The listing builds one solid part. Answer for the finished solid, in the listing's coordinates (mm). A direction names the side the tool comes from. Give positions to 0.01 mm unless a question says otherwise; leave off trailing zeros. Write each loop counter-clockwise with the first axis right and the second up, starting at its lowest first coordinate (ties: lowest second). Pieces come first, ordered by that corner, then holes.
```python
from build123d import *

# Parameters (mm, degrees)
BASPROSKE_W         = 3.175
BASPROSKE_H         = 5.291666667
TOOTHCUT_DEPTH      = 9.129212583
TEETHCUTS_COUNT     = 18
TEETHCUTS_ANGLE     = 340
SKETCH2_R           = 2
CUT_EXTRUDE3_DEPTH  = 9.090468526
SKETCH2_3_R         = 3.175
SKETCH2_3_R_2       = 2
BOSS_EXTRUDE1_DEPTH = 17.4625


with BuildPart() as part:
    # BasProSke → Base-Revolve (revolve)
    with BuildSketch(Plane(origin=(0, 0, 0), x_dir=(1, 0, 0), z_dir=(0, 1, 0)), mode=Mode.PRIVATE) as base_revolve_sk:
        with Locations((1.5875, 2.645833334)):
            Rectangle(BASPROSKE_W, BASPROSKE_H)
    revolve(base_revolve_sk.sketch.rotate(Axis((-10, 0, 0), (1, 0, 0)), 180), axis=Axis((-10, 0, 0), (1, 0, 0)))

    # TooCutSke → ToothCut (cut, through all)
    with BuildSketch(Plane(origin=(0, 0, 0), x_dir=(0, 0, -1), z_dir=(1, 0, 0))):
        with BuildLine():
            ThreePointArc((0.270003318, 4.067748898), (0, 4.0767), (-0.270003318, 4.067748898))
            ThreePointArc((-0.270003318, 4.067748898), (-0.437425956, 4.709129954), (-0.814487039, 5.254313352))
            ThreePointArc((-0.814487039, 5.254313352), (0, 5.317066667), (0.814487039, 5.254313352))
            ThreePointArc((0.814487039, 5.254313352), (0.437425956, 4.709129954), (0.270003318, 4.067748898))
        make_face()
    toothcut = extrude(amount=TOOTHCUT_DEPTH, mode=Mode.SUBTRACT)

    # TeethCuts: ToothCut ×18 about axis
    teethcuts_axis = Axis((-10, 0, 0), (1, 0, 0))
    for i in range(1, TEETHCUTS_COUNT):
        add(toothcut.rotate(teethcuts_axis, i * TEETHCUTS_ANGLE / (TEETHCUTS_COUNT - 1)), mode=Mode.SUBTRACT)

    # Sketch2 → Cut-Extrude3 (cut, through all)
    with BuildSketch(Plane.ZY):
        Circle(SKETCH2_R)
    extrude(amount=-CUT_EXTRUDE3_DEPTH, mode=Mode.SUBTRACT)

    # Sketch2_3 → Boss-Extrude1 (add)
    with BuildSketch(Plane.ZY):
        with Locations(Location((0, 0, 0), (0, 0, 180))):
            Circle(SKETCH2_3_R)
        Circle(SKETCH2_3_R_2, mode=Mode.SUBTRACT)
    extrude(amount=BOSS_EXTRUDE1_DEPTH)


solid = part.part
```
Item 1: Each of these flat-tipped pins is pushed along its axis until it touches: P1, Ø6, axis at x = -3.5, y = -3, coming from the -Z side (3 decimals); P2, Ø1.5, axis at x = -7.5, y = -2.5, coming from the +Z side; P3, Ø1, axis at x = -1.5, y = 3, coming from the +Z side; P4, Ø3, axis at y = 0, z = 0, coming from the -X side. Where does it stop, or does it pass through?
Conclusion:
P1: stops at z = -3.175
P2: stops at z = 2.65
P3: stops at z = 1.96
P4: passes through
Item 2: A cutting plane is placed at A-A, the plane z = 0. Give the vertices of the cut face in (x, y) (1 decimal), plus the area to 3 significant figures.
Conclusion:
outline: (-17.5, -3.2) - (0, -3.2) - (0, -4.1) - (3.2, -4.1) - (3.2, -2) - (-17.5, -2) - close; (-17.5, 2) - (3.2, 2) - (3.2, 4.1) - (0, 4.1) - (0, 3.2) - (-17.5, 3.2) - close
area: 54.2 mm2
Item 3: Consider probe 1 along Y at (x, z) = (1.9, 0); probe 2 along X at (y, z) = (-2.75, -3.25) (3 decimals); probe 3 along Z at (x, y) = (-10.75, -1.25). Determine where each line is inside the solid, lowest interval first.
Conclusion:
probe 1: y = -4.08 to -2, 2 to 4.08
probe 2: x = 0 to 3.175
probe 3: z = -2.92 to -1.56, 1.56 to 2.92
Item 4: A cutting plane is placed at C-C, the plane z = -4.5. Give the vertices of the cut face in (x, y) (3 decimals).
Conclusion:
outline: (0, -1.984) - (3.175, -1.984) - (3.175, -1.208) - (0, -1.208) - close; (0, -0.43) - (3.175, -0.43) - (3.175, 0.43) - (0, 0.43) - close; (0, 1.208) - (3.175, 1.208) - (3.175, 1.984) - (0, 1.984) - close
Item 5: A cutting plane is placed at B-B, the plane y = -2.5. Give the vertices of the cut face in (x, z) (1 decimal), plus the area to 3 significant figures.
Conclusion:
outline: (-17.5, -2) - (0, -2) - (0, -3.7) - (3.2, -3.7) - (3.2, 3.7) - (0, 3.7) - (0, 2) - (-17.5, 2) - close
area: 91.6 mm2
Item 6: A cutting plane is placed at D-D, the plane x = -1. Give the vertices of the cut face in (y, z) (3 decimals), plus the area to 3 significant figures.
Conclusion:
outline: circle Ø6.35 at (0, 0); hole circle Ø4 at (0, 0)
area: 19.1 mm2
Item 7: Which of the six approach directions +Z, -Z, +X, -X, +Y, -Y give full straight-line access (tool end or side, diameter ignored) to faces 1 (the face through (0, -3.12, -1.15)), 2 (the face through (1.565, -4.271, 2.017)), 3 (the face through (1.565, -2.713, 3.845)), 4 (the face through (1.565, 1.973, 4.272)), 5 (the face through (1.565, -1.245, -4.556))?
Conclusion:
face 1: -X
face 2: +X, -X, -Y
face 3: +Z, +X, -X
face 4: +X, -X
face 5: -Z, +X, -X
Item 8: Determine the mould class of faces 6 (the face through (1.57, 4.55, -1.2)), 7 (the face through (1.565, -4.258, -2.004)), 8 (the face through (1.565, 3.323, -3.356)) for opening direction Y: pulls with the +Y half, pulls with the -Y half, needs draft (parallel to the pull), parting line crosses it, or undercut.
Conclusion:
face 6: undercut
face 7: pulls with the -Y half
face 8: pulls with the +Y half
